Can you work these out from the model? Positions are in its coordinate system, mm. A direction names the side the tool comes from. Coordinates: 2 decimals unless noted, no trailing zeros. Order: outer loops, then holes, each group sorted by start corner. A loop starts at its lowest first (then second) coordinate and runs counter-clockwise, first axis right, second up. Notation, with made-up numbers: (10, 78.5) - (58, 78.5) arc R10 cw to (58, 91.5) - close; hole circle Ø4 at (-32, 1.25). An arc over 180 degrees is marked (long way). Use a Markdown table: item, result. Add a question column.
(1) For pin 1 Ø0.6 at (x, z) = (7, 0.5) entering from +Y; pin 2 Ø0.6 at (y, z) = (-40.5, 1) entering from +X, each with a flat end and sliding along its axis, tell me the tip position at first contact or that it passes through.
(2) I want a section at C-C (y = 34). List the corners of the cut face in (x, z) for me.
(3) On a 3-axis mill with a long thin cutter (end or side, diameter ignored), from which of +Z, -Z, +X, -X, +Y, -Y can I reach the whole of each face in a straight line? I mean faces 1 (the flat face through (-0.5, -41, 1)), 2 (the flat face through (-4.35, 32, 1)), 3 (the flat face through (4.35, 32, 1)). Say none if no direction works.
(4) If I drill on L1, parallel to Y at x = 1, z = 1.3; L2, parallel to X at y = 26.5, z = 0.8; L3, parallel to Y at x = 3, z = 0.15, over which ranges is the centre line in solid material (lowest first)? Write a range as [from, to].
(5) I want a section at D-D (x = 15). List the corners of the cut face in (y, z) for me.
(6) I want a section at A-A (x = 10.5). List the corners of the cut face in (y, z) for me.
(7) We'd pull the mould along Y, two halves only. Please class faces 4 (the cylindrical face through (-21.9, -46.6, 1)), 5 (the flat face through (0, -11, 0)), 6 (the flat face through (11, -42.171, 1)): pulls with the +Y half, pulls with the -Y half, needs draft (parallel to the pull), parting line crosses it, or undercut.
(8) I want a section at B-B (z = 1.25). List the corners of the cut face in (x, y) for me, and give its area (3 significant figures).
```python
from build123d import *

# Parameters (mm, degrees)
SALIENTE_EXTRUIR1_DEPTH = 2
CROQUIS3_W              = 23
CROQUIS3_H              = 3.3
CORTAR_EXTRUIR2_DEPTH   = 2
REDONDEO1_R             = 2
REDONDEO2_R             = 6
REDONDEO3_R             = 0.5


with BuildPart() as part:
    # Croquis1 → Saliente-Extruir1 (new body)
    with BuildSketch(Plane.XY):
        Polygon((-4.35, 20), (-22.5, 0.828732436), (-22.5, -47.171267564), (22.5, -47.171267564), (22.5, 0.828732436), (4.35, 19.999005159), (4.35, 45), (-4.35, 45), align=None)
    extrude(amount=SALIENTE_EXTRUIR1_DEPTH)

    # Croquis3 → Cortar-Extruir2 (cut)
    with BuildSketch(Plane.XY.offset(2)):
        with Locations((11, -40.521267564)):
            Rectangle(CROQUIS3_W, CROQUIS3_H)
    extrude(amount=-CORTAR_EXTRUIR2_DEPTH, mode=Mode.SUBTRACT)

    # Redondeo1
    redondeo1_edges = [part.edges().sort_by_distance(p)[0] for p in [
        (-4.35, 45, 1),
        (-4.35, 20, 1),
        (-22.5, -47.171267564, 1),
        (4.35, 19.999005159, 1),
        (4.35, 45, 1),
    ]]
    fillet(redondeo1_edges, radius=REDONDEO1_R)

    # Redondeo2
    redondeo2_edges = [part.edges().sort_by_distance(p)[0] for p in [
        (-22.5, 0.828732436, 1),
        (22.5, 0.828732436, 1),
    ]]
    fillet(redondeo2_edges, radius=REDONDEO2_R)

    # Redondeo3
    redondeo3_edges = [part.edges().sort_by_distance(p)[0] for p in [
        (22.5, -47.171267564, 1),
        (-0.5, -38.871267564, 1),
        (-0.5, -42.171267564, 1),
        (22.5, -42.171267564, 1),
        (22.5, -38.871267564, 1),
    ]]
    fillet(redondeo3_edges, radius=REDONDEO3_R)


solid = part.part
```
Answers follow:
| question | item | result |
|---|---|---|
| 1 | pin 1 | stops at y = 17.52 |
| 1 | pin 2 | stops at x = -0.5 |
| 2 | outline | (-4.35, 0) - (4.35, 0) - (4.35, 2) - (-4.35, 2) - close |
| 3 | face 1 | +Z, -Z, +X |
| 3 | face 2 | +Z, -Z, -X, +Y |
| 3 | face 3 | +Z, -Z, +X, +Y |
| 4 | L1 | y = [-47.17, -42.17], [-38.87, 45] |
| 4 | L2 | x = [-4.35, 4.35] |
| 4 | L3 | y = [-47.17, -42.17], [-38.87, 44.89] |
| 5 | outline | (-47.17, 0) - (-42.17, 0) - (-42.17, 2) - (-47.17, 2) - close; (-38.87, 0) - (8.75, 0) - (8.75, 2) - (-38.87, 2) - close |
| 6 | outline | (-47.17, 0) - (-42.17, 0) - (-42.17, 2) - (-47.17, 2) - close; (-38.87, 0) - (13.5, 0) - (13.5, 2) - (-38.87, 2) - close |
| 7 | face 4 | pulls with the -Y half |
| 7 | face 5 | needs draft |
| 7 | face 6 | undercut |
| 8 | outline | (-22.5, -45.17) arc R2 ccw to (-20.5, -47.17) - (22, -47.17) arc R0.5 ccw to (22.5, -46.67) - (22.5, -42.67) arc R0.5 ccw to (22, -42.17) - (0, -42.17) arc R0.5 cw to (-0.5, -41.67) - (-0.5, -39.37) arc R0.5 cw to (0, -38.87) - (22, -38.87) arc R0.5 ccw to (22.5, -38.37) - (22.5, -1.56) arc R6 ccw to (20.86, 2.56) - (4.9, 19.42) arc R2 cw to (4.35, 20.8) - (4.35, 43) arc R2 ccw to (2.35, 45) - (-2.35, 45) arc R2 ccw to (-4.35, 43) - (-4.35, 20.8) arc R2 cw to (-4.9, 19.42) - (-20.86, 2.56) arc R6 ccw to (-22.5, -1.56) - close |
| 8 | area | 2,810 mm² |
